from build123d import *

# Parameters (mm, degrees)
SKETCH1_R           = 60
SKETCH1_R_2         = 2.1
SKETCH1_R_3         = 3.1
BOSS_EXTRUDE1_DEPTH = 6
CUT_EXTRUDE1_DEPTH  = 3
SKETCH3_R           = 4.8
CUT_EXTRUDE2_DEPTH  = 3
SKETCH4_R           = 60
SKETCH4_R_2         = 55
BOSS_EXTRUDE2_DEPTH = 17
SKETCH5_W           = 25
SKETCH5_H           = 35
CUT_EXTRUDE3_DEPTH  = 87.539008545
FILLET1_R           = 2


with BuildPart() as part:
    # Sketch1 → Boss-Extrude1 (new body)
    with BuildSketch(Plane(origin=(0, 0, 0), x_dir=(1, 0, 0), z_dir=(0, 1, 0))):
        with Locations(Location((0, 0, 0), (0, 0, 270))):
            Circle(SKETCH1_R)
        with Locations(Location((-48, 0, 0), (0, 0, 270))):
            Circle(SKETCH1_R_2, mode=Mode.SUBTRACT)
        with Locations(Location((0, 0, 0), (0, 0, 270))):
            Circle(SKETCH1_R_3, mode=Mode.SUBTRACT)
        with Locations(Location((48, 0, 0), (0, 0, 90))):
            Circle(SKETCH1_R_2, mode=Mode.SUBTRACT)
    extrude(amount=BOSS_EXTRUDE1_DEPTH)

    # Sketch2 → Cut-Extrude1 (cut)
    with BuildSketch(Plane(origin=(0, 6, 0), x_dir=(1, 0, 0), z_dir=(0, 1, 0))):
        Polygon((-51.8, 2.193931023), (-51.8, -2.193931023), (-48, -4.387862046), (-44.2, -2.193931023), (-44.2, 2.193931023), (-48, 4.387862046), align=None)
        Polygon((48, 4.387862046), (51.8, 2.193931023), (51.8, -2.193931023), (48, -4.387862046), (44.2, -2.193931023), (44.2, 2.193931023), align=None)
    extrude(amount=-CUT_EXTRUDE1_DEPTH, mode=Mode.SUBTRACT)

    # Sketch3 → Cut-Extrude2 (cut)
    with BuildSketch(Plane.XZ):
        with Locations(Location((0, 0, 0), (0, 0, 270))):
            Circle(SKETCH3_R)
    extrude(amount=-CUT_EXTRUDE2_DEPTH, mode=Mode.SUBTRACT)

    # Sketch4 → Boss-Extrude2 (add)
    with BuildSketch(Plane(origin=(0, 6, 0), x_dir=(1, 0, 0), z_dir=(0, 1, 0))):
        with Locations(Location((0, 0, 0), (0, 0, 270))):
            Circle(SKETCH4_R)
        with Locations(Location((0, 0, 0), (0, 0, 270))):
            Circle(SKETCH4_R_2, mode=Mode.SUBTRACT)
    extrude(amount=BOSS_EXTRUDE2_DEPTH)

    # Sketch5 → Cut-Extrude3 (cut, through all)
    with BuildSketch(Plane(origin=(0, 6, 0), x_dir=(1, 0, 0), z_dir=(0, 1, 0))):
        with Locations((0, -50)):
            Rectangle(SKETCH5_W, SKETCH5_H)
    extrude(amount=CUT_EXTRUDE3_DEPTH, mode=Mode.SUBTRACT)

    # Fillet1
    # the kernel refuses this fillet: 2 mm, written as the material it takes off along each edge
    with BuildSketch(Plane(origin=(0, 23, 0), x_dir=(0.12573543795396686, 0, 0.9920638082515278), z_dir=(-0.9920638082515278, 0, 0.12573543795396686))) as fillet1_piece_1:
        with BuildLine():
            CenterArc((60 - FILLET1_R, -FILLET1_R), FILLET1_R, 0, 90)
            Line((60 - FILLET1_R, 0), (60, 0))
            Line((60, 0), (60, -FILLET1_R))
        make_face()
    revolve(axis=Axis((0, 23, 0), (0, 1, 0)), revolution_arc=345.553543265, mode=Mode.SUBTRACT)
    with BuildSketch(Plane(origin=(-12.5, 29.420959094, 58.683472972), x_dir=(-0.973374835212885, 0, -0.2292191749707888), z_dir=(0, -1, 0))) as fillet1_piece_2:
        with BuildLine():
            CenterArc((2.525577244, 1.999541851), FILLET1_R, 166.748894317, 104.477512186)
            Line((0.578827573, 2.457980201), (0, 0))
            ThreePointArc((0, 0), (1.284191819, -0.013744479), (2.568383638, 0))
        make_face()
    extrude(amount=23.420959094, mode=Mode.SUBTRACT)
    with BuildSketch(Plane(origin=(12.5, 29.420959094, 58.683472972), x_dir=(0.9733748352128844, 0, -0.22921917497079108), z_dir=(0, -1, 0))) as fillet1_piece_3:
        with BuildLine():
            CenterArc((2.525577244, -1.999541851), FILLET1_R, 88.773593497, 104.477512186)
            Line((0.578827573, -2.457980201), (0, 0))
            ThreePointArc((0, 0), (1.284191819, 0.013744479), (2.568383638, 0))
        make_face()
    extrude(amount=23.420959094, mode=Mode.SUBTRACT)
    with BuildSketch(Plane(origin=(0, 6, 0), x_dir=(0.2890214661785548, 0, 0.9573226165133667), z_dir=(0.9573226165133667, 0, -0.2890214661785548))) as fillet1_piece_4_section:
        with BuildLine():
            CenterArc((60 - FILLET1_R, FILLET1_R), FILLET1_R, 270, 90)
            Line((60 - FILLET1_R, 0), (60, 0))
            Line((60, 0), (60, FILLET1_R))
        make_face()
    fillet1_piece_4 = revolve(axis=Axis((0, 6, 0), (0, -1, 0)), revolution_arc=16.799381702, mode=Mode.PRIVATE)
    fillet1_piece_4 = split(fillet1_piece_4, bisect_by=Plane(origin=(12.5, 5.547238018, 59.104221097), z_dir=(-1, 0, 0)), keep=Keep.TOP, mode=Mode.PRIVATE)
    add(fillet1_piece_4, mode=Mode.SUBTRACT)
    with BuildSketch(Plane(origin=(0, 6, 0), x_dir=(0, 0, 1), z_dir=(1, 0, 0))) as fillet1_piece_5_section:
        with BuildLine():
            CenterArc((60 - FILLET1_R, FILLET1_R), FILLET1_R, 270, 90)
            Line((60 - FILLET1_R, 0), (60, 0))
            Line((60, 0), (60, FILLET1_R))
        make_face()
    fillet1_piece_5 = revolve(axis=Axis((0, 6, 0), (0, -1, 0)), revolution_arc=16.799381702, mode=Mode.PRIVATE)
    fillet1_piece_5 = split(fillet1_piece_5, bisect_by=Plane(origin=(-12.5, 5.5472381, 59.104220547), z_dir=(1, 0, 0)), keep=Keep.TOP, mode=Mode.PRIVATE)
    add(fillet1_piece_5, mode=Mode.SUBTRACT)
    with BuildSketch(Plane(origin=(0, 6, 0), x_dir=(0, 0, 1), z_dir=(1, 0, 0))) as fillet1_piece_6a_section:
        with BuildLine():
            CenterArc((60 - FILLET1_R, FILLET1_R), FILLET1_R, 270, 90)
            Line((60 - FILLET1_R, 0), (60, 0))
            Line((60, 0), (60, FILLET1_R))
        make_face()
    fillet1_piece_6a = revolve(axis=Axis((0, 6, 0), (0, -1, 0)), revolution_arc=16.799381702, mode=Mode.PRIVATE)
    fillet1_piece_6a = split(fillet1_piece_6a, bisect_by=Plane(origin=(-12.5, 5.540518873, 57.656474574), z_dir=(-1, 0, 0)), keep=Keep.TOP, mode=Mode.PRIVATE)
    with BuildSketch(Plane(origin=(-12.5, 29.420959094, 58.683472972), x_dir=(-0.973374835212885, 0, -0.2292191749707888), z_dir=(0, -1, 0))) as fillet1_piece_6b_section:
        with BuildLine():
            CenterArc((2.525577244, 1.999541851), FILLET1_R, 166.748894317, 104.477512186)
            Line((0.578827573, 2.457980201), (0, 0))
            ThreePointArc((0, 0), (1.284191819, -0.013744479), (2.568383638, 0))
        make_face()
    fillet1_piece_6b = extrude(amount=29.841918188, mode=Mode.PRIVATE)
    fillet1_piece_6b = split(fillet1_piece_6b, bisect_by=Plane(origin=(-13.085266846, 6, 57.965433437), z_dir=(0, -1, 0)), keep=Keep.TOP, mode=Mode.PRIVATE)
    fillet1_piece_6 = fillet1_piece_6a & fillet1_piece_6b
    add(fillet1_piece_6, mode=Mode.SUBTRACT)
    with BuildSketch(Plane(origin=(12.5, 29.420959094, 58.683472972), x_dir=(0.9733748352128844, 0, -0.22921917497079108), z_dir=(0, -1, 0))) as fillet1_piece_7a_section:
        with BuildLine():
            CenterArc((2.525577244, -1.999541851), FILLET1_R, 88.773593497, 104.477512186)
            Line((0.578827573, -2.457980201), (0, 0))
            ThreePointArc((0, 0), (1.284191819, 0.013744479), (2.568383638, 0))
        make_face()
    fillet1_piece_7a = extrude(amount=29.841918188, mode=Mode.PRIVATE)
    fillet1_piece_7a = split(fillet1_piece_7a, bisect_by=Plane(origin=(13.085266846, 6, 57.965433437), z_dir=(0, -1, 0)), keep=Keep.TOP, mode=Mode.PRIVATE)
    with BuildSketch(Plane(origin=(0, 6, 0), x_dir=(0.2890214661785548, 0, 0.9573226165133667), z_dir=(0.9573226165133667, 0, -0.2890214661785548))) as fillet1_piece_7b_section:
        with BuildLine():
            CenterArc((60 - FILLET1_R, FILLET1_R), FILLET1_R, 270, 90)
            Line((60 - FILLET1_R, 0), (60, 0))
            Line((60, 0), (60, FILLET1_R))
        make_face()
    fillet1_piece_7b = revolve(axis=Axis((0, 6, 0), (0, -1, 0)), revolution_arc=16.799381702, mode=Mode.PRIVATE)
    fillet1_piece_7b = split(fillet1_piece_7b, bisect_by=Plane(origin=(12.5, 5.540518947, 57.656474329), z_dir=(1, 0, 0)), keep=Keep.TOP, mode=Mode.PRIVATE)
    fillet1_piece_7 = fillet1_piece_7a & fillet1_piece_7b
    add(fillet1_piece_7, mode=Mode.SUBTRACT)


solid = part.part
Source: CAD feature listing. Evaluate the final solid. Frame: model axes, mm. A direction names the side the tool comes from. Round coordinates to 2 decimals unless told otherwise and drop trailing zeros. Loops run counter-clockwise (first coordinate to the right, second up) from the corner with the lowest first, then second, coordinate; pieces in that order, holes last. Notation, with made-up numbers: M 37,10 L 65,10 A20 cw 65,41 Z; hole C -10,79.5 d4. An arc over 180 degrees is marked long. Answer as CSV lines item,"result".
Q1. Line query: line 1 along X through (y, z) = (0.9, 0); line 2 along Y through (x, z) = (-16, 4.5); line 3 along Z through (x, y) = (-48, 10). Output: solid intervals per line, ascending.
Verdict:
line 1,"x = -60 to -50.1, -45.9 to -4.8, 4.8 to 45.9, 50.1 to 60"
line 2,"y = 0 to 6"
line 3,"z = -36 to -26.85, 26.85 to 36"
Q2. Cut plane B-B (y = 11). Return the cut outline in (x, z), plus the area to 3 significant figures.
Verdict:
outline,"M -15,58.09 A60 ccw long 15,58.09 A2 ccw 12.5,56.16 L 12.5,53.56 A55 cw long -12.5,53.56 L -12.5,56.16 A2 ccw Z"
area,"1,680 mm^2"
Q3. Reachability of faces 4 (the face through (4.05, 1.48, -2.58)), 5 (the face through (-12.5, 14, 55)), 6 (the face through (-34.1, 23, -43.4)), 7 (the face through (-50, 3, 2)) from +Z, -Z, +X, -X, +Y, -Y: full face, straight path, thin tool, end or side. Return the list, or none.
Verdict:
face 4,"-Y"
face 5,"+Z, +Y"
face 6,"+Z, -Z, +X, -X, +Y"
face 7,"+Y"
Q4. Contact query for flat-ended pins moving along their axis: pin 1 (8 mm diameter, centred on x = 12, y = 20, fed in from +Z); pin 2 (3 mm diameter, centred on x = 39, z = -10.5, fed in from -Y); pin 3 (7.5 mm diameter, centred on x = 0, z = 0, fed in from +Y); pin 4 (0.8 mm diameter, centred on y = 12.5, z = 55, fed in from -X). Output: stop coordinate, or through.
Verdict:
pin 1,"stops at z = 58.16"
pin 2,"stops at y = 0"
pin 3,"stops at y = 6"
pin 4,"stops at x = -24.88"
Q5. Cut plane A-A (z = 0). Count the separate pieces of the cut face and the enclosed holes in it, plus the area to 3 significant figures.
Verdict:
separate pieces,"4"
enclosed holes,"0"
area,"770 mm^2"
Q6. Pull-direction query (Z, two-part tool) for faces 1 (the face through (1, 0, 12)), 2 (the face through (2.64, 10.35, -59.94)), 3 (the face through (-50.05, 1.48, -0.46)); classes: +Z half, -Z half, draft (parallel to the pull), parting line (faces both ways), or undercut.
Verdict:
face 1,"draft"
face 2,"parting line"
face 3,"undercut"
